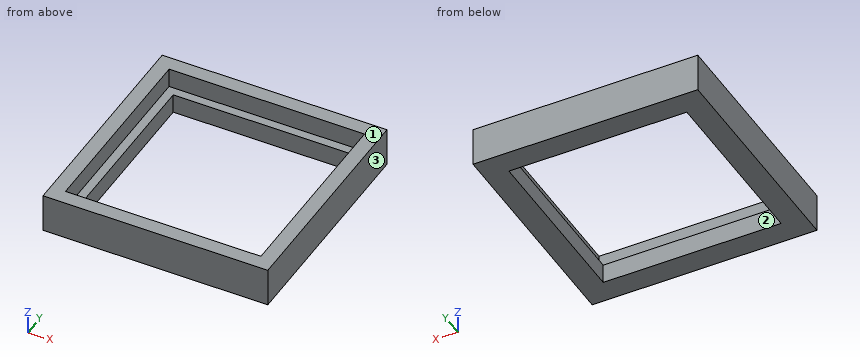
from build123d import *

# Parameters (mm, degrees)
SKETCH_1_W      = 11.5
SKETCH_1_H      = 11.5
SKETCH_1_W_2    = 10
SKETCH_1_H_2    = 10
EXTRUDE_1_DEPTH = 1
SKETCH_2_W      = 11.5
SKETCH_2_H      = 11.5
SKETCH_2_W_2    = 9.1
SKETCH_2_H_2    = 9.1
EXTRUDE_2_DEPTH = 1


with BuildPart() as part:
    # 草图1 → 凸台-拉伸1 (new body)
    with BuildSketch(Plane.XY):
        Rectangle(SKETCH_1_W, SKETCH_1_H)
        Rectangle(SKETCH_1_W_2, SKETCH_1_H_2, mode=Mode.SUBTRACT)
    extrude(amount=EXTRUDE_1_DEPTH)

    # 草图2 → 凸台-拉伸2 (add)
    with BuildSketch(Plane(origin=(0, 0, 0), x_dir=(-1, 0, 0), z_dir=(0, 0, -1))):
        Rectangle(SKETCH_2_W, SKETCH_2_H)
        Rectangle(SKETCH_2_W_2, SKETCH_2_H_2, mode=Mode.SUBTRACT)
    extrude(amount=EXTRUDE_2_DEPTH)


solid = part.part
Verification items for the finished model (mm, model axes). Face numbers are marked on the shaded views. Coordinates: 2 decimals unless noted, no trailing zeros. Order: outer loops, then holes, each group sorted by start corner. A loop starts at its lowest first (then second) coordinate and runs counter-clockwise, first axis right, second up. Notation, with made-up numbers: (-25.5, -9) -> (13.5, -9) arc R8 ccw to (13.5, -1) -> close; hole circle Ø1 at (-11.75, -20). An arc over 180 degrees is marked (long way). Put each result on its own line as item: value. Start each with the question number.
1. Cross-section at B-B, the plane y = -1.75. Record the boundary of the cut face in (x, z).
2. Material ranges on L1, parallel to X at y = -3, z = -0.15; L2, parallel to Y at x = 2, z = 0.05, recorded low to high. Write a range as [from, to].
3. Mould release check, pull along X, two halves, no side actions. Record for the marked faces 1, 2 and 3: released by +X, released by -X, zero draft, split by the parting line, or undercut.
4. Cross-section at A-A, the plane z = -0.75. Record the boundary of the cut face in (x, y).
Computed:
1. outline: (-5.75, -1) -> (-4.55, -1) -> (-4.55, 0) -> (-5, 0) -> (-5, 1) -> (-5.75, 1) -> close; (4.55, -1) -> (5.75, -1) -> (5.75, 1) -> (5, 1) -> (5, 0) -> (4.55, 0) -> close
2. L1: [-5.75, -4.55], [4.55, 5.75]
2. L2: [-5.75, -5], [5, 5.75]
3. face 1: zero draft
3. face 2: undercut
3. face 3: released by +X
4. outline: (-5.75, -5.75) -> (5.75, -5.75) -> (5.75, 5.75) -> (-5.75, 5.75) -> close; hole (-4.55, -4.55) -> (4.55, -4.55) -> (4.55, 4.55) -> (-4.55, 4.55) -> close
